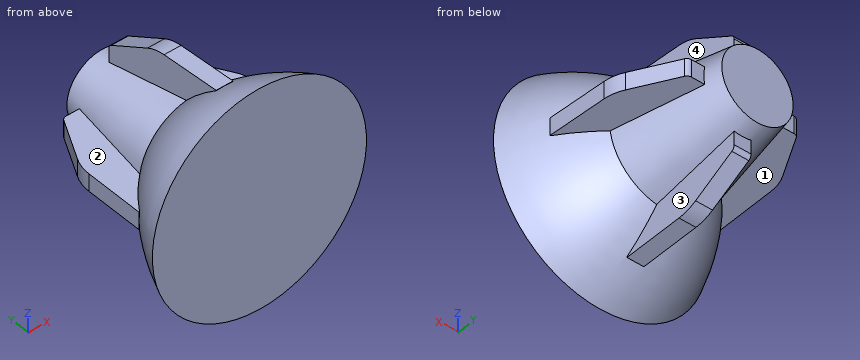
```python
from build123d import *

# Parameters (mm, degrees)
EXTRUDE7_DEPTH    = 5.08
CIRPATTERN1_COUNT = 4


with BuildPart() as part:
    # Sketch9 → Revolve3 (revolve)
    with BuildSketch(Plane.XY, mode=Mode.PRIVATE) as revolve3_sk:
        with BuildLine():
            Line((161.142350377, 194.292434626), (182.533079755, 194.292434626))
            Line((182.533079755, 194.292434626), (194.511888207, 130.975875666))
            ThreePointArc((194.511888207, 130.975875666), (212.420274366, 110.575127951), (225.334809451, 86.698034626))
            Line((225.334809451, 86.698034626), (161.142350377, 86.698034626))
            Line((161.142350377, 86.698034626), (161.142350377, 194.292434626))
        make_face()
    revolve(revolve3_sk.sketch.rotate(Axis((161.142350377, 86.698034626, 0), (0, 1, 0)), 90), axis=Axis((161.142350377, 86.698034626, 0), (0, 1, 0)))

    # Sketch10 → Extrude7 (add, symmetric)
    with BuildSketch(Plane.XY):
        with BuildLine():
            Line((161.142350377, 110.575127951), (161.142350377, 184.160379168))
            Line((161.142350377, 184.160379168), (191.859109399, 184.160379168))
            ThreePointArc((191.859109399, 184.160379168), (193.479127486, 183.715977344), (194.645640696, 182.507176898))
            Line((194.645640696, 182.507176898), (208.216170429, 157.658469957))
            ThreePointArc((208.216170429, 157.658469957), (210.434241625, 152.147730999), (211.311680607, 146.272513171))
            Line((211.311680607, 146.272513171), (212.420274366, 110.575127951))
            Line((212.420274366, 110.575127951), (161.142350377, 110.575127951))
        make_face()
    extrude7 = extrude(amount=EXTRUDE7_DEPTH, both=True)

    # CirPattern1: Extrude7 ×4 about axis
    cirpattern1_axis = Axis((161.142350377, 0, 0), (0, 1, 0))
    for i in range(1, CIRPATTERN1_COUNT):
        add(extrude7.rotate(cirpattern1_axis, i * 360 / CIRPATTERN1_COUNT))


solid = part.part
```
For this review, take the finished solid that the model builds, in its own axes (mm). Face numbers are marked on the shaded views. A direction names the side the tool comes from. Coordinates: 2 decimals unless noted, no trailing zeros. Answer as a JSON object with one key per item and string values. Group by question number.
1. Clearance check with flat-ended pins moving along their axes: P1, Ø1, axis at y = 107.5, z = -11, coming from the -X side; P2, Ø23, axis at x = 193, y = 137.5, coming from the -Z side; P3, Ø4, axis at x = 188, z = 0, coming from the +Y side; P4, Ø5, axis at x = 120.5, y = 177, coming from the -Z side. State where each tip first meets the part, or that it passes through.
2. For probe 1 along X at (y, z) = (174.5, -27.5); probe 2 along X at (y, z) = (105.5, 43.5); probe 3 along Y at (x, z) = (160.5, 29), list the stretches that pass through material, from the lowest coordinate up.
3. For the marked faces 1, 2, 3 and 4, list the 3-axis set-ups (+Z, -Z, +X, -X, +Y, -Y) from which the entire face can be reached by the end or side of a thin tool; tool diameter is ignored.
Final values:
{
 "1": {"P1": "x = 108.59", "P2": "z = -26.27", "P3": "y = 184.16", "P4": "through"},
 "2": {"probe 1": "156.06 to 166.22", "probe 2": "128.1 to 194.18", "probe 3": "86.7 to 184.16"},
 "3": {"face 1": "-Z, -X, +Y", "face 2": "+Z, -X, +Y", "face 3": "-Z, +X, +Y", "face 4": "+Z, +X, +Y"}
}
